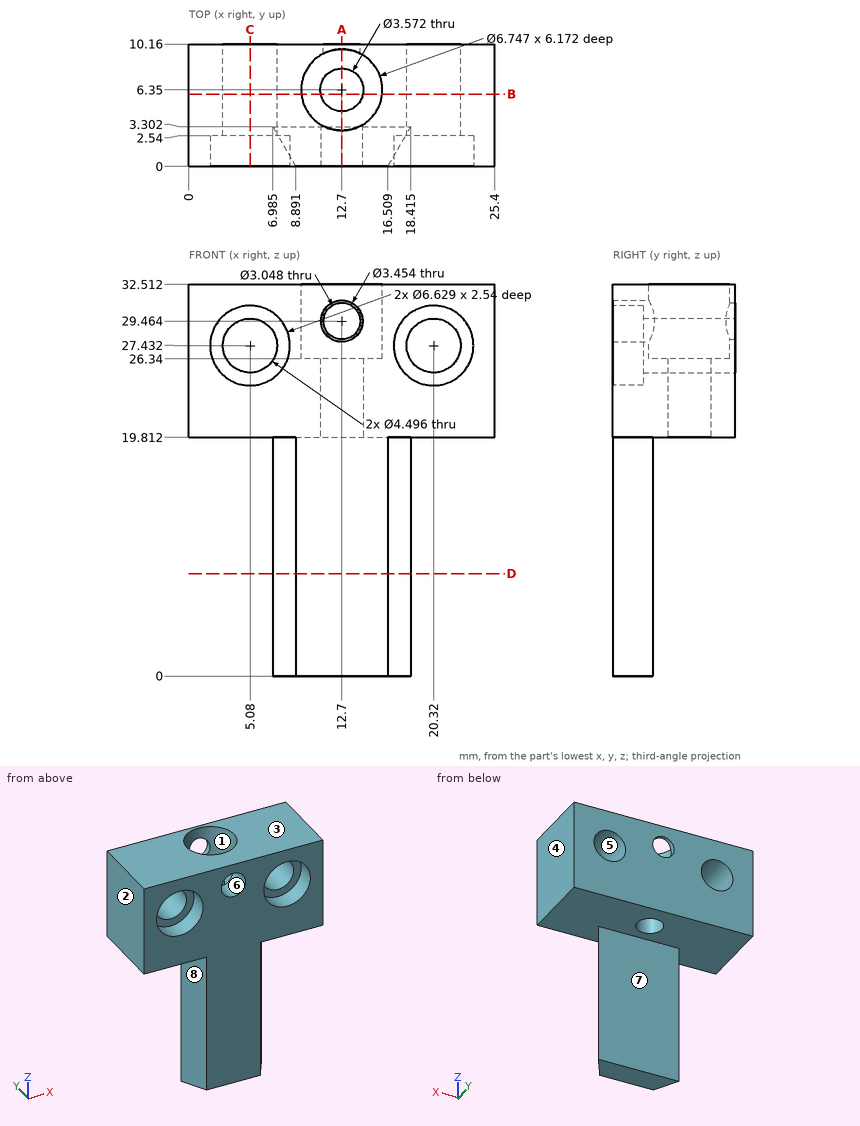
Could you check a few things on this drawing? It's one solid part, dimensions in mm from its lowest x, y, z. A direction names the side the tool comes from. Give positions to 0.01 mm unless a question says otherwise; leave off trailing zeros. Loops run counter-clockwise (first coordinate to the right, second up) from the corner with the lowest first, then second, coordinate; pieces in that order, holes last. Notation, with made-up numbers: M -24.5,-10 L 31.5,-10 A29 cw 31.5,20 Z; hole C -23,-33.5 d10. An arc over 180 degrees is marked long. Return JSON: item names as keys, results as strings.
Item 1: Imagine slicing it at C-C on x = 5.08. List the corners of the cut face in (y, z) for me.
A:
{"outline": "M 0,19.81 L 10.16,19.81 L 10.16,25.18 L 2.54,25.18 L 2.54,24.12 L 0,24.12 Z; M 0,30.75 L 2.54,30.75 L 2.54,29.68 L 10.16,29.68 L 10.16,32.51 L 0,32.51 Z"}
Item 2: I'm going to push flat-ended pins straight in: pin 1 Ø4 at (x, y) = (12.7, 6.35) entering from -Z; pin 2 Ø3.5 at (x, y) = (13.5, 5) entering from +Z; pin 3 Ø5 at (x, z) = (12.5, 5.5) entering from +Y. Where does each tip first touch, or does it pass through?
A:
{"pin 1": "stops at z = 19.81", "pin 2": "stops at z = 26.34", "pin 3": "stops at y = 3.3"}
Item 3: Please list where these lines run through material, in increasing order: line 1 (Z direction, x = 20.32, y = 7.25); line 2 (Z direction, x = 5.08, y = 0.8); line 3 (Z direction, x = 12.7, y = 9.6).
A:
{"line 1": "z = 19.81 to 25.18, 29.68 to 32.51", "line 2": "z = 19.81 to 24.12, 30.75 to 32.51", "line 3": "z = 19.81 to 26.34"}
Item 4: Thinking about a two-plate mould opening in X: for the marked faces 1, 2 and 3, which applies, released by +X, released by -X, zero draft, split by the parting line, or undercut?
A:
{"face 1": "undercut", "face 2": "released by -X", "face 3": "zero draft"}
Item 5: On a 3-axis mill with a long thin cutter (end or side, diameter ignored), from which of +Z, -Z, +X, -X, +Y, -Y can I reach the whole of each face in a straight line? I mean the marked faces 4, 5, 6, 7 and 8. Say none if no direction works.
A:
{"face 4": "+Z, -Z, +X, +Y, -Y", "face 5": "+Y, -Y", "face 6": "-Y", "face 7": "-Z, +X, -X, +Y", "face 8": "-Z, -X, -Y"}
Item 6: Imagine slicing it at A-A on x = 12.7. List the corners of the cut face in (y, z) for me, then the cut area to 3 significant figures.
A:
{"outline": "M 0,0 L 3.3,0 L 3.3,19.81 L 4.56,19.81 L 4.56,26.34 L 2.98,26.34 L 2.98,27.74 L 0,27.74 Z; M 0,31.19 L 2.98,31.19 L 2.98,32.51 L 0,32.51 Z; M 8.14,19.81 L 10.16,19.81 L 10.16,27.94 L 9.72,27.94 L 9.72,26.34 L 8.14,26.34 Z; M 9.72,30.99 L 10.16,30.99 L 10.16,32.51 L 9.72,32.51 Z", "area": "118 mm^2"}
Item 7: Imagine slicing it at B-B on y = 6. List the corners of the cut face in (x, z) for me (1 decimal).
A:
{"outline": "M 0,19.8 L 10.9,19.8 L 10.9,26.3 L 9.3,26.3 L 9.3,32.5 L 0,32.5 Z; M 14.5,19.8 L 25.4,19.8 L 25.4,32.5 L 16.1,32.5 L 16.1,26.3 L 14.5,26.3 Z; hole C 5.1,27.4 d4.5; hole C 20.3,27.4 d4.5"}
Item 8: Imagine slicing it at D-D on z = 8.5. List the corners of the cut face in (x, y) for me (1 decimal).
A:
{"outline": "M 7,3.3 L 8.9,0 L 16.5,0 L 18.4,3.3 Z"}
